Input: part model. Units: mm. Frame: model coordinates. Give positions to 0.01 mm unless a question says otherwise; leave off trailing zeros. Use a Markdown table: item, result. Add a question column.
1. Section query A-A, the plane z = 384.5. Count the separate pieces of the cut face and the enclosed holes in it, plus the area to 3 significant figures.
2. Material intervals for probe 1 along Y at (x, z) = (6.75, 392); probe 2 along Y at (x, z) = (0, 207); probe 3 along Y at (x, z) = (9.25, 209), sorted ascending.
3. Pin query (flat end, axial travel): pin 1 (0.8 mm diameter, centred on y = 21, z = 154, fed in from +X); pin 2 (3 mm diameter, centred on x = 0.5, z = 161, fed in from -Y); pin 3 (1 mm diameter, centred on x = 2.5, z = 165.5, fed in from +Y). Return the tip coordinate at first contact, or that it passes through.
4. Mould query, pull axis X, two halves, no side actions, for faces 1 (the flat face through (-10, 10, 246)), 2 (the flat face through (10, -10, 246)), 3 (the flat face through (-2.4, 0.4, 500)). Classes: released by +X, released by -X, zero draft, split by the parting line, or undercut.
```python
from build123d import *

# Parameters (mm, degrees)
SKETCH1_R           = 2.1
BOSS_EXTRUDE1_DEPTH = 500


with BuildPart() as part:
    # Sketch1 → Boss-Extrude1 (new body)
    with BuildSketch(Plane.XY):
        with BuildLine():
            Line((4.58, -30), (9.5, -30))
            ThreePointArc((9.5, -30), (9.853553391, -29.853553391), (10, -29.5))
            Line((10, -29.5), (10, -24.58))
            Line((10, -24.58), (8.545, -23.125))
            Line((8.545, -23.125), (8.2, -23.125))
            Line((8.2, -23.125), (8.2, -25.5))
            Line((8.2, -25.5), (6.560660172, -25.5))
            Line((6.560660172, -25.5), (3.9, -22.839339828))
            Line((3.9, -22.839339828), (3.9, -20.21))
            Line((3.9, -20.21), (3.69, -20))
            Line((3.69, -20), (3.9, -19.79))
            Line((3.9, -19.79), (3.9, -17.160660172))
            Line((3.9, -17.160660172), (6.560660172, -14.5))
            Line((6.560660172, -14.5), (8.2, -14.5))
            Line((8.2, -14.5), (8.2, -16.875))
            Line((8.2, -16.875), (8.545, -16.875))
            Line((8.545, -16.875), (10, -15.42))
            Line((10, -15.42), (10, -4.58))
            Line((10, -4.58), (8.545, -3.125))
            Line((8.545, -3.125), (8.2, -3.125))
            Line((8.2, -3.125), (8.2, -5.5))
            Line((8.2, -5.5), (6.560660172, -5.5))
            Line((6.560660172, -5.5), (3.9, -2.839339828))
            Line((3.9, -2.839339828), (3.9, -0.21))
            Line((3.9, -0.21), (3.69, 0))
            Line((3.69, 0), (3.9, 0.21))
            Line((3.9, 0.21), (3.9, 2.839339828))
            Line((3.9, 2.839339828), (6.560660172, 5.5))
            Line((6.560660172, 5.5), (8.2, 5.5))
            Line((8.2, 5.5), (8.2, 3.125))
            Line((8.2, 3.125), (8.545, 3.125))
            Line((8.545, 3.125), (10, 4.58))
            Line((10, 4.58), (10, 15.42))
            Line((10, 15.42), (8.545, 16.875))
            Line((8.545, 16.875), (8.2, 16.875))
            Line((8.2, 16.875), (8.2, 14.5))
            Line((8.2, 14.5), (6.560660172, 14.5))
            Line((6.560660172, 14.5), (3.9, 17.160660172))
            Line((3.9, 17.160660172), (3.9, 19.79))
            Line((3.9, 19.79), (3.69, 20))
            Line((3.69, 20), (3.9, 20.21))
            Line((3.9, 20.21), (3.9, 22.839339828))
            Line((3.9, 22.839339828), (6.560660172, 25.5))
            Line((6.560660172, 25.5), (8.2, 25.5))
            Line((8.2, 25.5), (8.2, 23.125))
            Line((8.2, 23.125), (8.545, 23.125))
            Line((8.545, 23.125), (10, 24.58))
            Line((10, 24.58), (10, 29.5))
            ThreePointArc((10, 29.5), (9.853553391, 29.853553391), (9.5, 30))
            Line((9.5, 30), (4.58, 30))
            Line((4.58, 30), (3.125, 28.545))
            Line((3.125, 28.545), (3.125, 28.2))
            Line((3.125, 28.2), (5.5, 28.2))
            Line((5.5, 28.2), (5.5, 26.560660172))
            Line((5.5, 26.560660172), (2.839339828, 23.9))
            Line((2.839339828, 23.9), (0.21, 23.9))
            Line((0.21, 23.9), (0, 23.69))
            Line((0, 23.69), (-0.21, 23.9))
            Line((-0.21, 23.9), (-2.839339828, 23.9))
            Line((-2.839339828, 23.9), (-5.5, 26.560660172))
            Line((-5.5, 26.560660172), (-5.5, 28.2))
            Line((-5.5, 28.2), (-3.125, 28.2))
            Line((-3.125, 28.2), (-3.125, 28.545))
            Line((-3.125, 28.545), (-4.58, 30))
            Line((-4.58, 30), (-9.5, 30))
            ThreePointArc((-9.5, 30), (-9.853553391, 29.853553391), (-10, 29.5))
            Line((-10, 29.5), (-10, 24.58))
            Line((-10, 24.58), (-8.545, 23.125))
            Line((-8.545, 23.125), (-8.2, 23.125))
            Line((-8.2, 23.125), (-8.2, 25.5))
            Line((-8.2, 25.5), (-6.560660172, 25.5))
            Line((-6.560660172, 25.5), (-3.9, 22.839339828))
            Line((-3.9, 22.839339828), (-3.9, 20.21))
            Line((-3.9, 20.21), (-3.69, 20))
            Line((-3.69, 20), (-3.9, 19.79))
            Line((-3.9, 19.79), (-3.9, 17.160660172))
            Line((-3.9, 17.160660172), (-6.560660172, 14.5))
            Line((-6.560660172, 14.5), (-8.2, 14.5))
            Line((-8.2, 14.5), (-8.2, 16.875))
            Line((-8.2, 16.875), (-8.545, 16.875))
            Line((-8.545, 16.875), (-10, 15.42))
            Line((-10, 15.42), (-10, 4.58))
            Line((-10, 4.58), (-8.545, 3.125))
            Line((-8.545, 3.125), (-8.2, 3.125))
            Line((-8.2, 3.125), (-8.2, 5.5))
            Line((-8.2, 5.5), (-6.560660172, 5.5))
            Line((-6.560660172, 5.5), (-3.9, 2.839339828))
            Line((-3.9, 2.839339828), (-3.9, 0.21))
            Line((-3.9, 0.21), (-3.69, 0))
            Line((-3.69, 0), (-3.9, -0.21))
            Line((-3.9, -0.21), (-3.9, -2.839339828))
            Line((-3.9, -2.839339828), (-6.560660172, -5.5))
            Line((-6.560660172, -5.5), (-8.2, -5.5))
            Line((-8.2, -5.5), (-8.2, -3.125))
            Line((-8.2, -3.125), (-8.545, -3.125))
            Line((-8.545, -3.125), (-10, -4.58))
            Line((-10, -4.58), (-10, -15.42))
            Line((-10, -15.42), (-8.545, -16.875))
            Line((-8.545, -16.875), (-8.2, -16.875))
            Line((-8.2, -16.875), (-8.2, -14.5))
            Line((-8.2, -14.5), (-6.560660172, -14.5))
            Line((-6.560660172, -14.5), (-3.9, -17.160660172))
            Line((-3.9, -17.160660172), (-3.9, -19.79))
            Line((-3.9, -19.79), (-3.69, -20))
            Line((-3.69, -20), (-3.9, -20.21))
            Line((-3.9, -20.21), (-3.9, -22.839339828))
            Line((-3.9, -22.839339828), (-6.560660172, -25.5))
            Line((-6.560660172, -25.5), (-8.2, -25.5))
            Line((-8.2, -25.5), (-8.2, -23.125))
            Line((-8.2, -23.125), (-8.545, -23.125))
            Line((-8.545, -23.125), (-10, -24.58))
            Line((-10, -24.58), (-10, -29.5))
            ThreePointArc((-10, -29.5), (-9.853553391, -29.853553391), (-9.5, -30))
            Line((-9.5, -30), (-4.58, -30))
            Line((-4.58, -30), (-3.125, -28.545))
            Line((-3.125, -28.545), (-3.125, -28.2))
            Line((-3.125, -28.2), (-5.5, -28.2))
            Line((-5.5, -28.2), (-5.5, -26.560660172))
            Line((-5.5, -26.560660172), (-2.839339828, -23.9))
            Line((-2.839339828, -23.9), (-0.21, -23.9))
            Line((-0.21, -23.9), (0, -23.69))
            Line((0, -23.69), (0.21, -23.9))
            Line((0.21, -23.9), (2.839339828, -23.9))
            Line((2.839339828, -23.9), (5.5, -26.560660172))
            Line((5.5, -26.560660172), (5.5, -28.2))
            Line((5.5, -28.2), (3.125, -28.2))
            Line((3.125, -28.2), (3.125, -28.545))
            Line((3.125, -28.545), (4.58, -30))
        make_face()
        with Locations((0, -20)):
            Circle(SKETCH1_R, mode=Mode.SUBTRACT)
        Polygon((-6.239339828, -12.7), (-8.2, -12.7), (-8.2, -7.3), (-6.239339828, -7.3), (-2.839339828, -3.9), (2.839339828, -3.9), (6.239339828, -7.3), (8.2, -7.3), (8.2, -12.7), (6.239339828, -12.7), (2.839339828, -16.1), (-2.839339828, -16.1), align=None, mode=Mode.SUBTRACT)
        Polygon((-6.239339828, 7.3), (-8.2, 7.3), (-8.2, 12.7), (-6.239339828, 12.7), (-2.839339828, 16.1), (2.839339828, 16.1), (6.239339828, 12.7), (8.2, 12.7), (8.2, 7.3), (6.239339828, 7.3), (2.839339828, 3.9), (-2.839339828, 3.9), align=None, mode=Mode.SUBTRACT)
        with Locations((0, 20)):
            Circle(SKETCH1_R, mode=Mode.SUBTRACT)
        Circle(SKETCH1_R, mode=Mode.SUBTRACT)
    extrude(amount=BOSS_EXTRUDE1_DEPTH)


solid = part.part
```
Result sheet:
| question | item | result |
|---|---|---|
| 1 | separate pieces | 1 |
| 1 | enclosed holes | 5 |
| 1 | area | 429 mm² |
| 2 | probe 1 | y = -30 to -25.5, -14.5 to -12.7, -7.3 to -5.5, 5.5 to 7.3, 12.7 to 14.5, 25.5 to 30 |
| 2 | probe 2 | y = -23.69 to -22.1, -17.9 to -16.1, -3.9 to -2.1, 2.1 to 3.9, 16.1 to 17.9, 22.1 to 23.69 |
| 2 | probe 3 | y = -30 to -23.83, -16.17 to -3.83, 3.83 to 16.17, 23.83 to 30 |
| 3 | pin 1 | stops at x = 3.9 |
| 3 | pin 2 | stops at y = -23.9 |
| 3 | pin 3 | stops at y = 24.06 |
| 4 | face 1 | released by -X |
| 4 | face 2 | released by +X |
| 4 | face 3 | zero draft |
